Read the model definition and answer for the solid it produces. Units are mm, in the model's axes. Round coordinates to 2 decimals unless told otherwise and drop trailing zeros. Loops run counter-clockwise (first coordinate to the right, second up) from the corner with the lowest first, then second, coordinate; pieces in that order, holes last. Notation, with made-up numbers: (36.25, -40) - (81.25, -40) arc R24 ccw to (81.25, -22) - close; hole circle Ø5 at (-7.75, 27.5). An arc over 180 degrees is marked (long way). Use one line per item in the form item = value. Start each with the question number.
```python
from build123d import *

# Parameters (mm, degrees)
F0_W     = 229
F0_H     = 149
F0_W_2   = 220
F0_H_2   = 139
F1_DEPTH = 3.3
F3_W     = 5
F3_H     = 5
F3_R     = 1.5
F4_DEPTH = 0.1


# Not quite as in the source:
# - a feature names something its author has since deleted; it is built from what else it names


with BuildPart() as f1:
    # F0 (on Top) → F1 (new body)
    with BuildSketch(Plane.XY):
        with Locations((114.5, -74.5)):
            Rectangle(F0_W, F0_H)
        with Locations((114.5, -74.5)):
            Rectangle(F0_W_2, F0_H_2, mode=Mode.SUBTRACT)
    extrude(amount=F1_DEPTH)

    # F3 (on offset) → F4 (join)
    with BuildSketch(Plane.XY.offset(1.8)):
        with Locations((165.5, 2.5)):
            Rectangle(F3_W, F3_H)
        with Locations((165.5, 2.5)):
            Circle(F3_R, mode=Mode.SUBTRACT)
        with Locations((82.5, -151.5)):
            Rectangle(F3_W, F3_H)
        with Locations((82.5, -151.5)):
            Circle(F3_R, mode=Mode.SUBTRACT)
        with Locations((165.5, -151.5)):
            Rectangle(F3_W, F3_H)
        with Locations((165.5, -151.5)):
            Circle(F3_R, mode=Mode.SUBTRACT)
        with Locations((82.5, 2.5)):
            Rectangle(F3_W, F3_H)
        with Locations((82.5, 2.5)):
            Circle(F3_R, mode=Mode.SUBTRACT)
    extrude(amount=F4_DEPTH)


solid = f1.part
```
1) A cutting plane is placed at C-C on x = 139.5. Write down the section's boundary in (y, z).
2) Straight lines are drawn through the part: line 1 (Y direction, x = 106.5, z = 3.2); line 2 (X direction, y = -66.5, z = 1.5). For each, find the intervals that lie inside material, in ascending order. Write a range as from..to.
3) A cutting plane is placed at A-A on z = 0.6. Write down the section's boundary in (x, y).
4) Flat-ended cylindrical pins translate along their axes: pin 1 (2.5 mm diameter, centred on x = 82, y = -150.5, fed in from +Z); pin 2 (4 mm diameter, centred on x = 166, y = 1.5, fed in from +Z); pin 3 (2.5 mm diameter, centred on x = 165.5, y = 3.5, fed in from -Z). Find the tip coordinate at first contact, or state that the pin passes through.
5) A cutting plane is placed at B-B on y = -20.5. Write down the section's boundary in (x, z).
Checks:
q1.outline = (-149, 0) - (-144, 0) - (-144, 3.3) - (-149, 3.3) - close; (-5, 0) - (0, 0) - (0, 3.3) - (-5, 3.3) - close
q2.line_1 = -149..-144, -5..0
q2.line_2 = 0..4.5, 224.5..229
q3.outline = (0, -149) - (229, -149) - (229, 0) - (0, 0) - close; hole (4.5, -144) - (224.5, -144) - (224.5, -5) - (4.5, -5) - close
q4.pin_1 = 1.9
q4.pin_2 = 3.3
q4.pin_3 = 1.8
q5.outline = (0, 0) - (4.5, 0) - (4.5, 3.3) - (0, 3.3) - close; (224.5, 0) - (229, 0) - (229, 3.3) - (224.5, 3.3) - close
